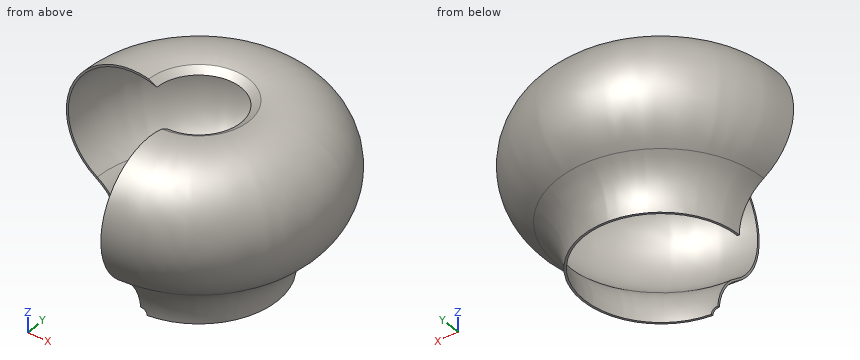
```python
from build123d import *

# Parameters (mm, degrees)
F1_ANGLE = 270
F3_DEPTH = 100.001


# Not quite as in the source:
# - a feature names something its author has since deleted; it is built from what else it names


with BuildPart() as f1:
    # F0 (on Right) → F1 (revolve)
    with BuildSketch(Plane.YZ):
        with BuildLine():
            ThreePointArc((-76.6564003216, 35.4822715112), (-92.9111910846, 98.6026476259), (-31.6640544802, 120.9003686165))
            Line((-31.6640544802, 120.9003686165), (-37.7450487886, 124.4749024837))
            ThreePointArc((-37.7450487886, 124.4749024837), (-95.7605829794, 96.1486735392), (-77.4808250738, 34.2291458878))
            ThreePointArc((-77.4808250738, 34.2291458878), (-63.9346767138, 19.4432539414), (-59.0274766756, 0))
            Line((-59.0274766756, 0), (-57.5274766756, 0))
            ThreePointArc((-57.5274766756, 0), (-62.6143288187, 20.1550695325), (-76.6564003216, 35.4822715112))
        make_face()
    revolve(axis=Axis((0, 0, 76), (0, 0, 1)), revolution_arc=F1_ANGLE)

    # F2 (on Front) → F3 (cut, through all)
    with BuildSketch(Plane.XZ):
        with BuildLine():
            Line((-4.5, 0), (4.5, 0))
            ThreePointArc((4.5, 0), (0, 4.5), (-4.5, 0))
        make_face()
    extrude(amount=F3_DEPTH, mode=Mode.SUBTRACT)


solid = f1.part
```
Model file for the job. Use its own axes, mm. Coordinates: 2 decimals unless noted, no trailing zeros. Write each loop counter-clockwise with the first axis right and the second up, starting at its lowest first coordinate (ties: lowest second). Pieces come first, ordered by that corner, then holes. Notation, with made-up numbers: (78, -1) - (109, -1) arc R34 cw to (109, 34) - close; hole circle Ø4 at (-27.5, 49). An arc over 180 degrees is marked (long way). One line per question, with ' | ' between items. Start each with the question number.
Q1. Pin check, flat tips, straight feed: pin 1 (1 mm diameter, centred on x = 51.5, z = 99, fed in from +Y); pin 2 (1 mm diameter, centred on x = 52, y = -77, fed in from +Z); pin 3 (6 mm diameter, centred on y = 36.5, z = 31.5, fed in from +X); pin 4 (10 mm diameter, centred on x = -20.5, y = 47, fed in from +Z). Stop position of each tip, or through.
Q2. Cut at A-A, the plane z = 52. List the corners of the cut face in (x, y).
Q3. Cut at B-B, the plane z = 18.5. List the corners of the cut face in (x, y), then the cut area to 3 significant figures.
Q4. Drill centre lines: line 1 (X direction, y = 21, z = 116); line 2 (X direction, y = 4.5, z = 21); line 3 (Z direction, x = -39, y = 58). Where is each one in solid material? Low to high. Write a range as [from, to].
Answer below:
1) pin 1: y = 79.55 | pin 2: z = 102.48 | pin 3: x = 69.04 | pin 4: z = 126
2) outline: (-93.86, 0) - (-92.15, 0) arc R92.15 cw (long way) to (0, -92.15) - (0, -93.86) arc R93.86 ccw (long way) to start
3) outline: (-63.44, 0) - (-61.77, 0) arc R61.77 cw (long way) to (0, -61.77) - (0, -63.44) arc R63.44 ccw (long way) to start | area: 494 mm^2
4) line 1: [-77.19, -74.52], [74.52, 77.19] | line 2: [-64.66, -62.92], [62.92, 64.66] | line 3: [27.79, 29.96], [120.23, 121.87]
